Verification items for this drawing (mm, ordinates from the low corner). Round coordinates to 2 decimals unless told otherwise and drop trailing zeros. Order: outer loops, then holes, each group sorted by start corner. A loop starts at its lowest first (then second) coordinate and runs counter-clockwise, first axis right, second up. Notation, with made-up numbers: M 40.5,-30 L 97.5,-30 A24 ccw 97.5,-13 Z; hole C 49,66 d2. An arc over 180 degrees is marked long. Use CSV: the item, a comma, the result in double quotes. Start each with the question number.
Q1. Sectioned sample at B-B (x = 25.5). Enter the section's corners in (y, z), and give its area (4 significant figures).
Q2. Gauge pin test, flat ends, axial feed: pin 1 Ø1.5 at (y, z) = (58, 2) entering from +X; pin 2 Ø20 at (x, y) = (25, 45.5) entering from -Z; pin 3 Ø4 at (x, z) = (24, 2.5) entering from -Y. Record the tip position at first contact, or that the pin passes through.
Q3. Mould release check, pull along Z, two halves, no side actions. Record for the marked faces 1, 2 and 3: +Z half, -Z half, draft (parallel to the pull), parting line (faces both ways), or undercut.
Q4. Scan lines: line 1 (Y direction, x = 25.5, z = 9.7); line 2 (Z direction, x = 12, y = 16.5); line 3 (X direction, y = 50, z = 2.25). Record each from-to range of solid material in increasing order.
Q5. Sectioned sample at C-C (y = 81.5). Enter the section's corners in (x, z).
Q6. Sectioned sample at D-D (z = 2.5). Enter the section's corners in (x, y).
Q7. Sectioned sample at A-A (y = 23.8). Enter the section's corners in (x, z), and give its area (4 significant figures).
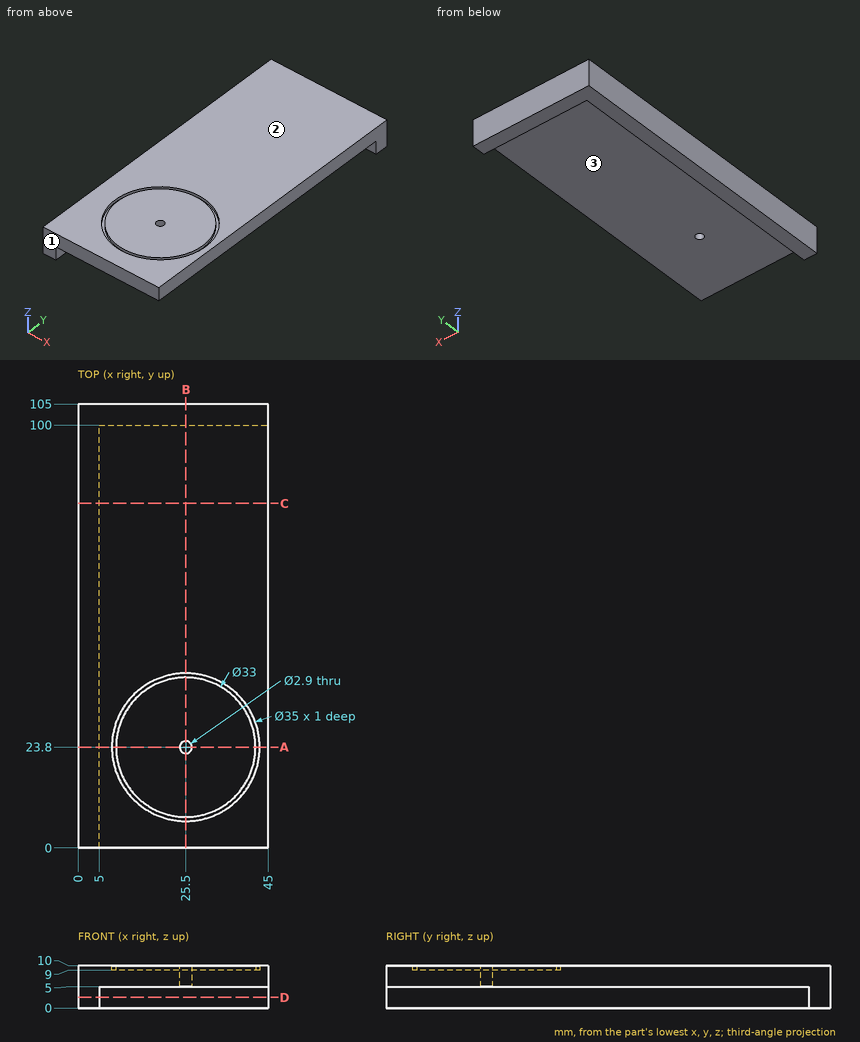
Verdict:
1,outline,"M 0,5 L 22.35,5 L 22.35,10 L 7.3,10 L 7.3,9 L 6.3,9 L 6.3,10 L 0,10 Z; M 25.25,5 L 100,5 L 100,0 L 105,0 L 105,10 L 41.3,10 L 41.3,9 L 40.3,9 L 40.3,10 L 25.25,10 Z"
1,area,"533.5 mm²"
2,pin 1,"stops at x = 5"
2,pin 2,"stops at z = 5"
2,pin 3,"stops at y = 100"
3,face 1,"draft"
3,face 2,"+Z half"
3,face 3,"-Z half"
4,line 1,"y = 0 to 6.3, 7.3 to 22.35, 25.25 to 40.3, 41.3 to 105"
4,line 2,"z = 5 to 10"
4,line 3,"x = 0 to 5"
5,outline,"M 0,0 L 5,0 L 5,5 L 45,5 L 45,10 L 0,10 Z"
6,outline,"M 0,0 L 5,0 L 5,100 L 45,100 L 45,105 L 0,105 Z"
7,outline,"M 0,0 L 5,0 L 5,5 L 24.05,5 L 24.05,10 L 9,10 L 9,9 L 8,9 L 8,10 L 0,10 Z; M 26.95,5 L 45,5 L 45,10 L 43,10 L 43,9 L 42,9 L 42,10 L 26.95,10 Z"
7,area,"233.5 mm²"
